Verification items for the finished model (mm, model axes). A direction names the side the tool comes from. Give positions to 0.01 mm unless a question says otherwise; leave off trailing zeros. Write each loop counter-clockwise with the first axis right and the second up, starting at its lowest first coordinate (ties: lowest second). Pieces come first, ordered by that corner, then holes. Notation, with made-up numbers: M 84.5,72.25 L 115.5,72.25 A21 ccw 115.5,77.25 Z; hole C 53.5,7 d4. An arc over 180 degrees is marked long. Answer as a JSON object with one key per item and string values.
```python
from build123d import *

# Parameters (mm, degrees)
BOSS_EXTRUDE1_DEPTH = 22.606
SKETCH2_W           = 32.636558609
SKETCH2_H           = 30.48
CUT_EXTRUDE1_DEPTH  = 6
CUT_EXTRUDE2_DEPTH  = 6
FILLET1_R           = 2


with BuildPart() as part:
    # Sketch1 → Boss-Extrude1 (new body, symmetric)
    with BuildSketch(Plane.XY):
        Polygon((0, 20.9042), (13.335, 20.9042), (13.335, 0), (30.335, 0), (30.335, 5), (18.335, 5), (18.335, 25.9042), (0, 25.9042), align=None)
    extrude(amount=BOSS_EXTRUDE1_DEPTH, both=True)

    # Sketch2 → Cut-Extrude1 (cut, through all)
    with BuildSketch(Plane.XZ.offset(-20.9042)):
        with Locations((16.318279305, 0)):
            Rectangle(SKETCH2_W, SKETCH2_H)
    extrude(amount=-CUT_EXTRUDE1_DEPTH, mode=Mode.SUBTRACT)

    # Sketch4 → CSK for #8 Flat Head Socket Cap Screw1 (revolve, cut)
    with BuildSketch(Plane(origin=(24.335, 5, 0), x_dir=(0, 0, 1), z_dir=(1, 0, 0))):
        Polygon((0, 0), (0, 5), (2.2479, 5), (2.2479, 2.658961536), (4.5593, 0), align=None)
    revolve(axis=Axis((24.335, 11.35, 0), (0, -1, 0)), mode=Mode.SUBTRACT)

    # Sketch5 → Cut-Extrude2 (cut, through all)
    with BuildSketch(Plane(origin=(0, 5, 0), x_dir=(1, 0, 0), z_dir=(0, 1, 0))):
        with BuildLine():
            Line((30.335, 22.606), (18.335, 22.606))
            Line((18.335, 22.606), (29.545282756, 2.975391336))
            ThreePointArc((29.545282756, 2.975391336), (30.134211001, 1.539204912), (30.335, 2.1e-08))
            Line((30.335, 2.1e-08), (30.335, 22.606))
        make_face()
        with BuildLine():
            Line((30.335, -22.606), (30.335, 2.1e-08))
            ThreePointArc((30.335, 2.1e-08), (30.134211007, -1.539204892), (29.545282756, -2.975391336))
            Line((29.545282756, -2.975391336), (18.335, -22.606))
            Line((18.335, -22.606), (30.335, -22.606))
        make_face()
    extrude(amount=-CUT_EXTRUDE2_DEPTH, mode=Mode.SUBTRACT)

    # Fillet1
    fillet1_edges = [part.edges().sort_by_distance(p)[0] for p in [
        (18.335, 25.9042, 18.923),
        (18.335, 25.9042, -18.923),
    ]]
    fillet(fillet1_edges, radius=FILLET1_R)

    # Mirror1: part across plane


with BuildPart() as part_1:
    add(part.part)
    add(part.part.mirror(Plane(origin=(0, 0, 0), x_dir=(0, 0, 1), z_dir=(1, 0, 0))))


solid = part_1.part
```
1) Section check C-C on y = 3.25. Record the boundary of the cut face in (x, z) (3 decimals), and give its area (3 significant figures).
Completed:
{"outline": "M -29.545,-2.975 L -18.335,-22.606 L -13.335,-22.606 L -13.335,22.606 L -18.335,22.606 L -29.545,2.975 A6 ccw Z; M 13.335,-22.606 L 18.335,-22.606 L 29.545,-2.975 A6 ccw 29.545,2.975 L 18.335,22.606 L 13.335,22.606 Z; hole C -24.335,0 d6.076; hole C 24.335,0 d6.076", "area": "974 mm2"}
2) Access from +Z, -Z, +X, -X, +Y, -Y to the whole of each face (thin tool, end or side, straight path). Record for faces 5 (the face through (-18.335, 14, 0)), 6 (the face through (0, 23, 15.24)), 7 (the face through (-20, 0, 0)), 8 (the face through (13.335, 11, 0)).
Completed:
{"face 5": "+Z, -Z, -X, +Y", "face 6": "+X, -X, +Y", "face 7": "+Z, -Z, +X, -X, -Y", "face 8": "+Z, -Z, -Y"}
3) Release check for a two-part mould opening along Z. For faces 1 (the face through (-21.96, 2.51, -0.31)), 2 (the face through (23.86, 2.54, -12.93)), 3 (the face through (0, 25.904, -19)), 4 (the face through (16, 20.904, 0)) record: pulls with the +Z half, pulls with the -Z half, needs draft (parallel to the pull), parting line crosses it, or undercut.
Completed:
{"face 1": "undercut", "face 2": "pulls with the -Z half", "face 3": "needs draft", "face 4": "undercut"}
4) Section check A-A on x = 8. Record the boundary of the cut face in (y, z).
Completed:
{"outline": "M 20.9,-22.61 L 25.9,-22.61 L 25.9,-15.24 L 20.9,-15.24 Z; M 20.9,15.24 L 25.9,15.24 L 25.9,22.61 L 20.9,22.61 Z"}
5) Thickness scan on L1, parallel to X at y = 1.95, z = 0 (3 decimals); L2, parallel to Z at x = 0, y = 23.25; L3, parallel to X at y = 9.5, z = 15 (3 decimals). Record the ranges inside material, lowest first.
Completed:
{"L1": "x = -30.335 to -26.583, -22.087 to -13.335, 13.335 to 22.087, 26.583 to 30.335", "L2": "z = -22.61 to -15.24, 15.24 to 22.61", "L3": "x = -18.335 to -13.335, 13.335 to 18.335"}
6) Section check B-B on y = 6.25. Record the boundary of the cut face in (x, z) (3 decimals).
Completed:
{"outline": "M -18.335,-22.606 L -13.335,-22.606 L -13.335,22.606 L -18.335,22.606 Z; M 13.335,-22.606 L 18.335,-22.606 L 18.335,22.606 L 13.335,22.606 Z"}
7) Section check D-D on z = -9. Record the boundary of the cut face in (x, y) (3 decimals).
Completed:
{"outline": "M -26.105,0 L -13.335,0 L -13.335,20.904 L -18.335,20.904 L -18.335,5 L -26.105,5 Z; M 13.335,0 L 26.105,0 L 26.105,5 L 18.335,5 L 18.335,20.904 L 13.335,20.904 Z"}
8) Go/stop test with flat-tipped pins: pin 1 (5.5 mm diameter, centred on y = 18.5, z = -8.5, fed in from +X) (3 decimals); pin 2 (4 mm diameter, centred on x = -24.335, z = 0, fed in from -Y); pin 3 (6 mm diameter, centred on x = 24.335, z = 0, fed in from +Y); pin 4 (13 mm diameter, centred on x = -25, z = 10.5, fed in from +Y). Record where each tip stops, or that it passes through.
Completed:
{"pin 1": "stops at x = 18.335", "pin 2": "passes through", "pin 3": "stops at y = 3.21", "pin 4": "stops at y = 5"}
